Job drawing, mm, ordinate dimensions from the low corner. One solid piece. A direction names the side the tool comes from. Coordinates: 2 decimals unless noted, no trailing zeros. Write each loop counter-clockwise with the first axis right and the second up, starting at its lowest first coordinate (ties: lowest second). Pieces come first, ordered by that corner, then holes. Notation, with made-up numbers: (52.5, -19) - (80.5, -19) arc R17 ccw to (80.5, -10) - close; hole circle Ø3 at (-29, 34). An arc over 180 degrees is marked (long way). Use a Markdown table: item, result.
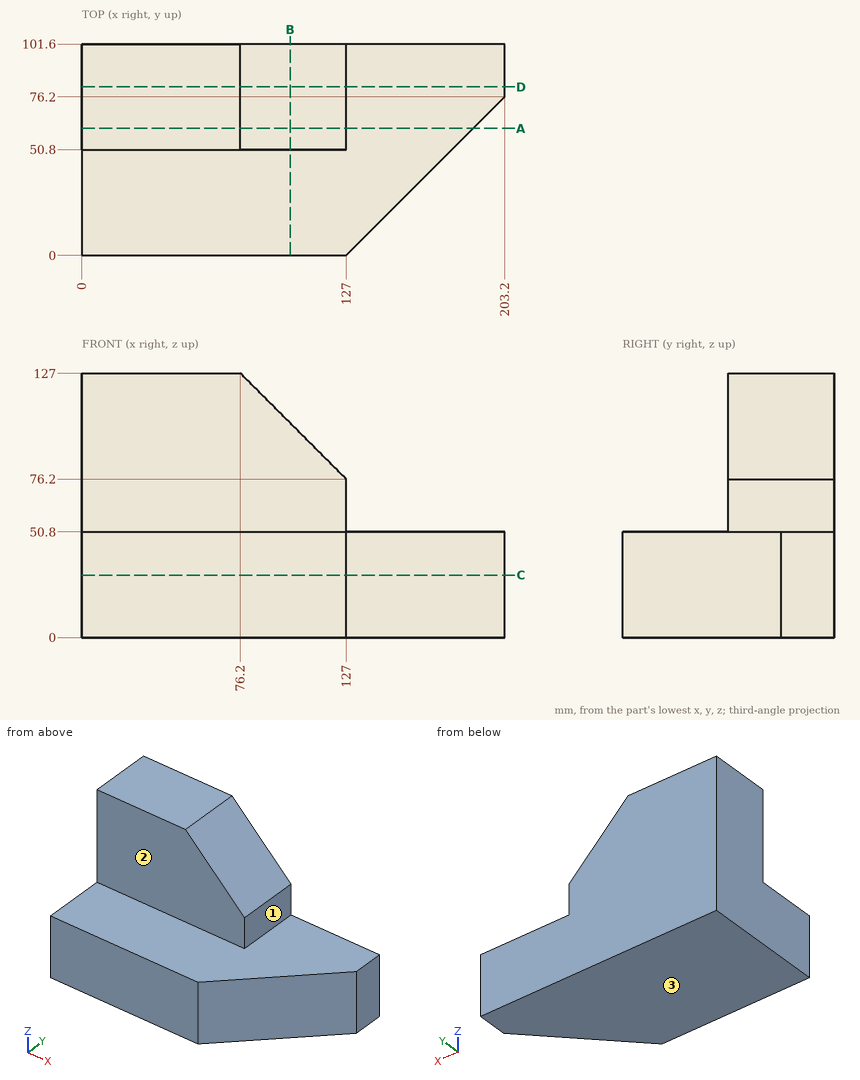
Item 1: Band-saw the part on D-D, the plane y = 81. Give the cut face in (x, z).
From the geometry:
| item | result |
|---|---|
| outline | (0, 0) - (203.2, 0) - (203.2, 50.8) - (127, 50.8) - (127, 76.2) - (76.2, 127) - (0, 127) - close |
Item 2: Which spindle directions (+Z, -Z, +X, -X, +Y, -Y) get a long thin tool onto all of the face, cutting with end or side? Do the marked faces 1, 2 and 3. Say none if no direction does.
From the geometry:
| item | result |
|---|---|
| face 1 | +Z, +X, +Y, -Y |
| face 2 | +Z, +X, -X, -Y |
| face 3 | -Z, +X, -X, +Y, -Y |
Item 3: Drill centre lines: probe 1 along X at (y, z) = (97, 68); probe 2 along Y at (x, z) = (47, 51.5); probe 3 along Z at (x, y) = (104.5, 42). Where is each one in solid material? Low to high.
From the geometry:
| item | result |
|---|---|
| probe 1 | 0 to 127 |
| probe 2 | 50.8 to 101.6 |
| probe 3 | 0 to 50.8 |
Item 4: Band-saw the part on C-C, the plane z = 30. Give the cut face in (x, y).
From the geometry:
| item | result |
|---|---|
| outline | (0, 0) - (127, 0) - (203.2, 76.2) - (203.2, 101.6) - (0, 101.6) - close |
Item 5: Band-saw the part on B-B, the plane x = 100. Give the cut face in (y, z).
From the geometry:
| item | result |
|---|---|
| outline | (0, 0) - (101.6, 0) - (101.6, 103.2) - (50.8, 103.2) - (50.8, 50.8) - (0, 50.8) - close |
Item 6: Drop flat-ended pins along their axis: P1, Ø5, axis at y = 46.5, z = 47.5, coming from the +X side; P2, Ø10, axis at x = 65.5, y = 14.5, coming from the +Z side; P3, Ø23, axis at x = 88, z = 99.5, coming from the -Y side. Give the stop position or say it passes through.
From the geometry:
| item | result |
|---|---|
| P1 | x = 176 |
| P2 | z = 50.8 |
| P3 | y = 50.8 |
Item 7: Band-saw the part on A-A, the plane y = 61. Give the cut face in (x, z), then the cut area to 3 significant figures.
From the geometry:
| item | result |
|---|---|
| outline | (0, 0) - (188, 0) - (188, 50.8) - (127, 50.8) - (127, 76.2) - (76.2, 127) - (0, 127) - close |
| area | 17,900 mm^2 |
